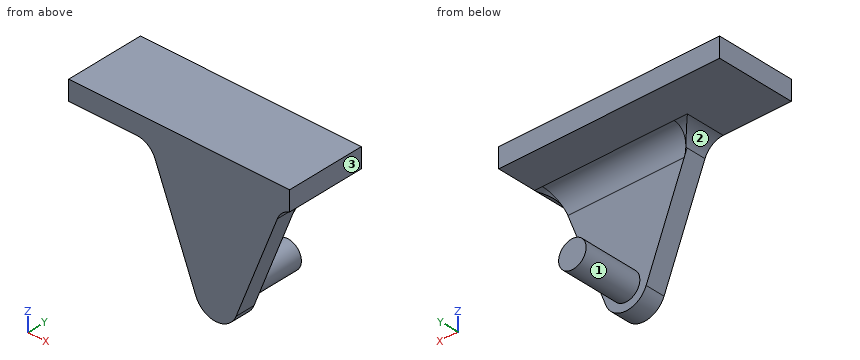
from build123d import *

# Parameters (mm, degrees)
SKETCH1_R           = 11
SKETCH1_R_2         = 7
BOSS_EXTRUDE1_DEPTH = 10
BOSS_EXTRUDE2_START = 10
SKETCH1_3_W         = 112.5
SKETCH1_3_H         = 10
SKETCH1_3_R         = 7
BOSS_EXTRUDE2_DEPTH = 30
FILLET1_R           = 10


with BuildPart() as part:
    # Sketch1 → Boss-Extrude1 (new body)
    # profile 1 of 6: a face of its own
    with BuildSketch(Plane(origin=(0, 0, 0), x_dir=(1, 0, 0), z_dir=(0, 1, 0))):
        Polygon((-37.5, -65), (-33.550296394, -55), (-75, -55), (-75, -65), align=None)
    # profile 2 of 6: a face of its own
    with BuildSketch(Plane(origin=(0, 0, 0), x_dir=(1, 0, 0), z_dir=(0, 1, 0))):
        Polygon((33.550296394, -55), (-33.550296394, -55), (-37.5, -65), (37.5, -65), align=None)
    # profile 3 of 6: a face of its own
    with BuildSketch(Plane(origin=(0, 0, 0), x_dir=(1, 0, 0), z_dir=(0, 1, 0))):
        Polygon((37.5, -55), (33.550296394, -55), (37.5, -65), align=None)
    # profile 4 of 6: a face of its own
    with BuildSketch(Plane(origin=(0, 0, 0), x_dir=(1, 0, 0), z_dir=(0, 1, 0))):
        with BuildLine():
            ThreePointArc((11, 0), (-2.056720175, -10.806012314), (-10.230891295, 4.040898824))
            Line((-10.230891295, 4.040898824), (-33.550296394, -55))
            Line((-33.550296394, -55), (33.550296394, -55))
            Line((33.550296394, -55), (10.230891295, 4.040898824))
            ThreePointArc((10.230891295, 4.040898824), (10.806012314, 2.056720175), (11, 0))
        make_face()
    # profile 5 of 6: a face of its own
    with BuildSketch(Plane(origin=(0, 0, 0), x_dir=(1, 0, 0), z_dir=(0, 1, 0))):
        Circle(SKETCH1_R)
        Circle(SKETCH1_R_2, mode=Mode.SUBTRACT)
    # profile 6 of 6: a face of its own
    with BuildSketch(Plane(origin=(0, 0, 0), x_dir=(1, 0, 0), z_dir=(0, 1, 0))):
        Circle(SKETCH1_R_2)
    extrude(amount=BOSS_EXTRUDE1_DEPTH)

    # Sketch1<3> → Boss-Extrude2 (add)
    with BuildSketch(Plane(origin=(0, 0, 0), x_dir=(1, 0, 0), z_dir=(0, 1, 0)).offset(BOSS_EXTRUDE2_START)):
        with Locations((-18.75, -60)):
            Rectangle(SKETCH1_3_W, SKETCH1_3_H)
        with Locations(Location((0, 0, 0), (0, 0, 270))):
            Circle(SKETCH1_3_R)
    extrude(amount=BOSS_EXTRUDE2_DEPTH)

    # Fillet1
    # the kernel refuses this fillet: 10 mm, written as the material it adds along each edge
    with BuildSketch(Plane(origin=(-33.550296394, 0, 55), x_dir=(-1, 0, 0), z_dir=(0, 1, 0))) as fillet1_piece_1:
        with BuildLine():
            CenterArc((FILLET1_R * 0.680204781295, -FILLET1_R), FILLET1_R, 90, 68.447449105)
            Line((-FILLET1_R * 0.249876245536, -FILLET1_R * 0.632645561443), (-FILLET1_R * 0.268477866073, -FILLET1_R * 0.625298472672))
            Line((-FILLET1_R * 0.268477866073, -FILLET1_R * 0.625298472672), (-FILLET1_R * 0.0136040956259, FILLET1_R * 0.02))
            Line((-FILLET1_R * 0.0136040956259, FILLET1_R * 0.02), (FILLET1_R * 0.680204781295, FILLET1_R * 0.02))
            Line((FILLET1_R * 0.680204781295, FILLET1_R * 0.02), (FILLET1_R * 0.680204781295, 0))
        make_face()
    extrude(amount=10)
    with BuildSketch(Plane(origin=(33.550296394, 0, 55), x_dir=(1, 0, 0), z_dir=(0, 1, 0))) as fillet1_piece_2:
        with BuildLine():
            CenterArc((6.988874819, 9.526984745), FILLET1_R, 201.552550895, 50.754421911)
            Line((-2.31193545, 5.85344036), (-2.497951655, 5.779969472))
            Line((-2.497951655, 5.779969472), (-0.186016205, -0.073470888))
            Line((-0.186016205, -0.073470888), (0, -0.2))
            ThreePointArc((0, -0.2), (1.974851803, -0.2), (3.888920182, -0.190539695))
            Line((3.888920182, -0.190539695), (3.949703606, 0))
        make_face()
    extrude(amount=10)
    with BuildSketch(Plane(origin=(58.550296394, 10, 55), x_dir=(0, 1, 0), z_dir=(-1, 0, 0))) as fillet1_piece_3_section:
        with BuildLine():
            CenterArc((FILLET1_R, FILLET1_R), FILLET1_R, 180, 90)
            Line((0, FILLET1_R), (-FILLET1_R * 0.02, FILLET1_R))
            Line((-FILLET1_R * 0.02, FILLET1_R), (-FILLET1_R * 0.02, -FILLET1_R * 0.02))
            Line((-FILLET1_R * 0.02, -FILLET1_R * 0.02), (FILLET1_R, -FILLET1_R * 0.02))
            Line((FILLET1_R, -FILLET1_R * 0.02), (FILLET1_R, 0))
        make_face()
    fillet1_piece_3 = extrude(amount=117.100592788, mode=Mode.PRIVATE)
    fillet1_piece_3 = split(fillet1_piece_3, bisect_by=Plane(origin=(28.268391296, 12.297159596, 41.627084904), z_dir=(-0.9300810268318512, 0, 0.3673544385568373)), keep=Keep.TOP, mode=Mode.PRIVATE)
    fillet1_piece_3 = split(fillet1_piece_3, bisect_by=Plane(origin=(-28.268391296, 12.297159596, 41.627084904), z_dir=(0.9300810268318513, 0, 0.36735443855683725)), keep=Keep.TOP, mode=Mode.PRIVATE)
    add(fillet1_piece_3)
    with BuildSketch(Plane(origin=(-33.550296394, 0, 55), x_dir=(-1, 0, 0), z_dir=(0, 1, 0))) as fillet1_piece_4a_section:
        with BuildLine():
            CenterArc((FILLET1_R * 0.680204781295, -FILLET1_R), FILLET1_R, 90, 68.447449105)
            Line((-FILLET1_R * 0.249876245536, -FILLET1_R * 0.632645561443), (-FILLET1_R * 0.268477866073, -FILLET1_R * 0.625298472672))
            Line((-FILLET1_R * 0.268477866073, -FILLET1_R * 0.625298472672), (-FILLET1_R * 0.0136040956259, FILLET1_R * 0.02))
            Line((-FILLET1_R * 0.0136040956259, FILLET1_R * 0.02), (FILLET1_R * 0.680204781295, FILLET1_R * 0.02))
            Line((FILLET1_R * 0.680204781295, FILLET1_R * 0.02), (FILLET1_R * 0.680204781295, 0))
        make_face()
    fillet1_piece_4a = extrude(amount=27.005119532, mode=Mode.PRIVATE)
    fillet1_piece_4a = split(fillet1_piece_4a, bisect_by=Plane(origin=(-34.492064323, 10, 53.615464114), z_dir=(0, 1, 0)), keep=Keep.TOP, mode=Mode.PRIVATE)
    with BuildSketch(Plane(origin=(58.550296394, 10, 55), x_dir=(0, 1, 0), z_dir=(-1, 0, 0))) as fillet1_piece_4b_section:
        with BuildLine():
            CenterArc((FILLET1_R, FILLET1_R), FILLET1_R, 180, 90)
            Line((0, FILLET1_R), (-FILLET1_R * 0.02, FILLET1_R))
            Line((-FILLET1_R * 0.02, FILLET1_R), (-FILLET1_R * 0.02, -FILLET1_R * 0.02))
            Line((-FILLET1_R * 0.02, -FILLET1_R * 0.02), (FILLET1_R, -FILLET1_R * 0.02))
            Line((FILLET1_R, -FILLET1_R * 0.02), (FILLET1_R, 0))
        make_face()
    fillet1_piece_4b = extrude(amount=117.100592788, mode=Mode.PRIVATE)
    fillet1_piece_4b = split(fillet1_piece_4b, bisect_by=Plane(origin=(-34.377193324, 12.222070762, 57.093567044), z_dir=(-0.9300810268318513, 0, -0.36735443855683725)), keep=Keep.TOP, mode=Mode.PRIVATE)
    fillet1_piece_4 = fillet1_piece_4a & fillet1_piece_4b
    add(fillet1_piece_4)
    with BuildSketch(Plane(origin=(58.550296394, 10, 55), x_dir=(0, 1, 0), z_dir=(-1, 0, 0))) as fillet1_piece_5a_section:
        with BuildLine():
            CenterArc((FILLET1_R, FILLET1_R), FILLET1_R, 180, 90)
            Line((0, FILLET1_R), (-FILLET1_R * 0.02, FILLET1_R))
            Line((-FILLET1_R * 0.02, FILLET1_R), (-FILLET1_R * 0.02, -FILLET1_R * 0.02))
            Line((-FILLET1_R * 0.02, -FILLET1_R * 0.02), (FILLET1_R, -FILLET1_R * 0.02))
            Line((FILLET1_R, -FILLET1_R * 0.02), (FILLET1_R, 0))
        make_face()
    fillet1_piece_5a = extrude(amount=117.100592788, mode=Mode.PRIVATE)
    fillet1_piece_5a = split(fillet1_piece_5a, bisect_by=Plane(origin=(37.5, 12.040069704, 52.357079342), z_dir=(-1, 0, 0)), keep=Keep.TOP, mode=Mode.PRIVATE)
    fillet1_piece_5a = split(fillet1_piece_5a, bisect_by=Plane(origin=(32.843361018, 12.040069704, 53.210155884), z_dir=(0.9300810268318512, 0, -0.3673544385568373)), keep=Keep.TOP, mode=Mode.PRIVATE)
    with BuildSketch(Plane(origin=(33.550296394, 0, 55), x_dir=(1, 0, 0), z_dir=(0, 1, 0))) as fillet1_piece_5b_section:
        with BuildLine():
            CenterArc((6.988874819, 9.526984745), FILLET1_R, 201.552550895, 50.754421911)
            Line((-2.31193545, 5.85344036), (-2.497951655, 5.779969472))
            Line((-2.497951655, 5.779969472), (-0.186016205, -0.073470888))
            Line((-0.186016205, -0.073470888), (0, -0.2))
            ThreePointArc((0, -0.2), (1.974851803, -0.2), (3.888920182, -0.190539695))
            Line((3.888920182, -0.190539695), (3.949703606, 0))
        make_face()
    fillet1_piece_5b = extrude(amount=25.733683924, mode=Mode.PRIVATE)
    fillet1_piece_5b = split(fillet1_piece_5b, bisect_by=Plane(origin=(33.943390061, 10, 53.584203188), z_dir=(0, 1, 0)), keep=Keep.TOP, mode=Mode.PRIVATE)
    fillet1_piece_5 = fillet1_piece_5a & fillet1_piece_5b
    add(fillet1_piece_5)


solid = part.part
Model file for the job. Use its own axes, mm. Face numbers are marked on the shaded views. Give positions to 0.01 mm unless a question says otherwise; leave off trailing zeros. Write each loop counter-clockwise with the first axis right and the second up, starting at its lowest first coordinate (ties: lowest second). Pieces come first, ordered by that corner, then holes. Notation, with made-up numbers: M -1,79 L 32,79 A34 cw 32,114 Z; hole C 24.25,-19.5 d5. An arc over 180 degrees is marked long. One line per item, written item: value. Start each with the question number.
Q1. Saw through at B-B, the plane x = 0. Write the cut outline in (y, z).
Q2. Drop flat-ended pins along their axis: pin 1 Ø8 at (y, z) = (5.5, 1) entering from +X; pin 2 Ø8 at (y, z) = (18, 0) entering from -X; pin 3 Ø4 at (x, z) = (-1, 47) entering from -Y; pin 4 Ø8 at (x, y) = (-2, 33.5) entering from -Z. Give the stop position or say it passes through.
Q3. Probe probe 1 along Y at (x, z) = (-5.5, 5.5); probe 2 along Z at (x, y) = (-60.5, 23.5); probe 3 along X at (y, z) = (18.5, -0.5). List the from-to ranges inside material, lowest first. Write a range as [from, to].
Q4. Saw through at C-C, the plane y = 16. Write the cut outline in (x, z), plus the area to 3 significant figures.
Q5. Saw through at A-A, the plane y = 3. Write the cut outline in (x, z).
Q6. Saw through at D-D, the plane z = 0. Write the cut outline in (x, y).
Q7. Two-plate mould, pull along Z, no slides. Class the marked faces 1, 2 and 3: +Z half, -Z half, draft (parallel to the pull), parting line (faces both ways), or undercut.
Output values:
1. outline: M 0,-11 L 10,-11 L 10,-7 L 40,-7 L 40,7 L 10,7 L 10,45 A10 cw 20,55 L 40,55 L 40,65 L 0,65 Z
2. pin 1: stops at x = 13.8
2. pin 2: stops at x = -7
2. pin 3: stops at y = 0
2. pin 4: stops at z = -7
3. probe 1: y = [0, 10]
3. probe 2: z = [55, 65]
3. probe 3: x = [-6.98, 6.98]
4. outline: M -75,55 L -40.35,55 A10 cw -36.35,54.17 L 35.59,54.17 A10 cw 37.5,55 L 37.5,65 L -75,65 Z; C 0,0 d14
4. area: 1,340 mm²
5. outline: M -75,55 L -40.35,55 A10 cw -31.05,48.67 L -10.23,-4.04 A11 ccw 10.23,-4.04 L 31.24,49.15 A10 cw 37.5,55 L 37.5,65 L -75,65 Z
6. outline: M -11.83,0 L 11.83,0 L 11.83,10 L 7,10 L 7,40 L -7,40 L -7,10 L -11.83,10 Z
7. face 1: undercut
7. face 2: -Z half
7. face 3: draft
